from build123d import *

# Parameters (mm, degrees)
F0_R     = 2.5
F1_DEPTH = 5
F2_W     = 2
F2_H     = 1
F3_DEPTH = 3
F4_R     = 0.5
F5_DEPTH = 25


with BuildPart() as f1:
    # F0 (on Top) → F1 (new body)
    with BuildSketch(Plane.XY):
        Circle(F0_R)
    extrude(amount=F1_DEPTH)

    # F2 (on face) → F3 (join)
    with BuildSketch(Plane.XY.offset(5)):
        with Locations((0, -1.5)):
            Rectangle(F2_W, F2_H)
    extrude(amount=F3_DEPTH)

    # F4 (on face) → F5 (cut)
    with BuildSketch(Plane.XY.offset(5)):
        Circle(F4_R)
    extrude(amount=-F5_DEPTH, mode=Mode.SUBTRACT)


solid = f1.part
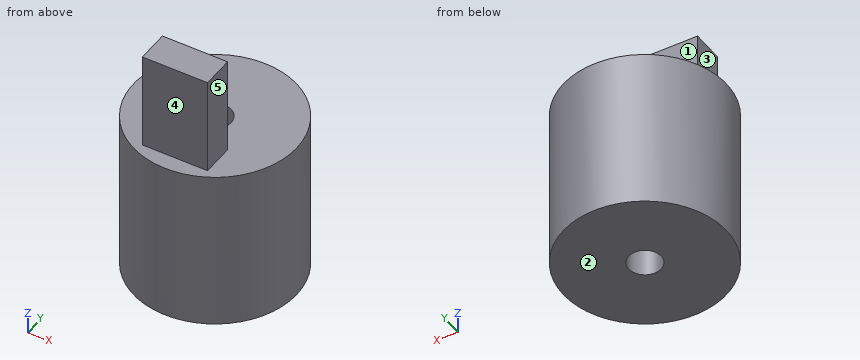
Check sheet for the modelled part. Datum: model origin and axes. Units: mm. Face numbers are marked on the shaded views. A direction names the side the tool comes from. Round coordinates to 2 decimals unless told otherwise and drop trailing zeros. Order: outer loops, then holes, each group sorted by start corner. A loop starts at its lowest first (then second) coordinate and runs counter-clockwise, first axis right, second up.
(1) Cross-section at D-D, the plane z = 2.5. Enter the section's corners in (x, y).
(2) Cross-section at A-A, the plane x = 0. Enter the section's corners in (y, z).
(3) Scan lines: probe 1 along Y at (x, z) = (0, 1.2); probe 2 along Z at (x, y) = (-1.5, -1.2); probe 3 along X at (y, z) = (-0.25, 4.25). Record each from-to range of solid material in increasing order.
(4) Access from +Z, -Z, +X, -X, +Y, -Y to the whole of each face (thin tool, end or side, straight path). Record for the marked faces 1, 2, 3, 4 and 5.
(5) Cross-section at C-C, the plane z = 6. Enter the section's corners in (x, y), and give its area (3 significant figures).
(6) Go/stop test with flat-tipped pins: P1, Ø1.5, axis at y = 1, z = 6, coming from the +X side; P2, Ø1.6, axis at x = 0, z = 7, coming from the +Y side; P3, Ø1, axis at x = 0.5, z = 6, coming from the -Y side; P4, Ø0.5, axis at y = -1.5, z = 7, coming from the -X side. Record where each tip stops, or that it passes through.
(7) Cross-section at B-B, the plane y = 0. Enter the section's corners in (x, z).
Check sheet entries:
1. outline: circle Ø5 at (0, 0); hole circle Ø1 at (0, 0)
2. outline: (-2.5, 0) - (-0.5, 0) - (-0.5, 5) - (-1, 5) - (-1, 8) - (-2, 8) - (-2, 5) - (-2.5, 5) - close; (0.5, 0) - (2.5, 0) - (2.5, 5) - (0.5, 5) - close
3. probe 1: y = -2.5 to -0.5, 0.5 to 2.5
3. probe 2: z = 0 to 5
3. probe 3: x = -2.49 to -0.43, 0.43 to 2.49
4. face 1: +Z, +X, -X, +Y
4. face 2: -Z, +X, -X, +Y, -Y
4. face 3: +Z, -X, +Y, -Y
4. face 4: +Z, +X, -X, -Y
4. face 5: +Z, +X, +Y, -Y
5. outline: (-1, -2) - (1, -2) - (1, -1) - (-1, -1) - close
5. area: 2.00 mm2
6. P1: passes through
6. P2: stops at y = -1
6. P3: stops at y = -2
6. P4: stops at x = -1
7. outline: (-2.5, 0) - (-0.5, 0) - (-0.5, 5) - (-2.5, 5) - close; (0.5, 0) - (2.5, 0) - (2.5, 5) - (0.5, 5) - close
